Can you work these out from the model? Positions are in its coordinate system, mm. A direction names the side the tool comes from. Give positions to 0.01 mm unless a question says otherwise; leave off trailing zeros. Loops run counter-clockwise (first coordinate to the right, second up) from the corner with the lowest first, then second, coordinate; pieces in that order, holes last. Notation, with made-up numbers: M 21,8.25 L 69,8.25 A26 cw 69,26.25 Z; hole C 48.25,-7.75 d7. An arc over 180 degrees is marked long. Answer as a JSON object with one key per item and string values.
Autodesk Fusion 360 part; units mm, degrees
sketch "Colour Sensor Servo Seat Outline" plane through (0, 0, 0) normal (0, 0, 1) x (1, 0, 0)
  line L0 (0, 0) -> (54.5, 0)
  line L1 (54.5, 0) -> (54.5, 39)
  line L2 (54.5, 39) -> (0, 39)
  line L3 (0, 39) -> (0, 0)
  dimension "d1" = 39
  dimension "d2" = 54.5
extrude "Extrude1" add sketch "Colour Sensor Servo Seat Outline" along normal blind 30
sketch "Colour Sensor Servo Hole" plane through (0, 0, 30) normal (0, 0, 1) x (-1, 0, 0)
  line L0 (0, -39) -> (0, 0)
  line L1 (0, 0) -> (-54.5, 0)
  line L2 (-54.5, 0) -> (-54.5, -39)
  line L3 (-54.5, -39) -> (0, -39)
  line L4 (-54.5, -8.5) -> (-18, -8.5)
  line L5 (-18, -8.5) -> (-18, -21.5)
  line L6 (-18, -21.5) -> (-54.5, -21.5)
  line L7 (-54.5, -21.5) -> (-54.5, -8.5)
  line L8 (-54.5, 0) -> (-18, 0)
  line L9 (-18, 0) -> (-18, -30)
  line L10 (-18, -30) -> (-54.5, -30)
  line L11 (-54.5, -30) -> (-54.5, 0)
  line L12 (-54.5, -21.5) -> (-49.8, -21.5)
  line L13 (-49.8, -21.5) -> (-49.8, -8.5)
  line L14 (-49.8, -8.5) -> (-54.5, -8.5)
  line L15 (-54.5, -8.5) -> (-54.5, -21.5)
  point P0 (-54.5, -21.5)
  point P1 (-54.5, -30)
  dimension "d6" = 13
  dimension "d8" = 36.5
  dimension "d9" = 30
  dimension "d10" = 8.5
  dimension "d11" = 8.5
  dimension "d12" = 4.7
extrude "Extrude2" cut sketch "Colour Sensor Servo Hole" against normal blind 5 contours L2 L4 L6 L7 L11 L12 L13 L14 L15
extrude "Extrude3" cut sketch "Colour Sensor Servo Hole" against normal blind 25.82 contours L4 L5 L6 L9 L13
chamfer "Chamfer1" distance 24 distance2 9 1 edges at (27.25, 39, 0) measured on face at (36.3333, 39, 20)
sketch "Front Ribs" plane through (0, 39, 0) normal (0, 1, 0) x (-1, 0, 0)
  line L0 (-54.5, 24) -> (0, 24)
  line L1 (0, 24) -> (0, 30)
  line L2 (0, 30) -> (-54.5, 30)
  line L3 (-54.5, 30) -> (-54.5, 24)
  line L4 (0, 0) -> (0, 24)
  line L5 (0, 24) -> (-54.5, 24)
  line L6 (-54.5, 24) -> (-54.5, 0)
  line L7 (-54.5, 0) -> (0, 0)
  line L8 (-46, 24) -> (-18, 24)
  line L9 (-18, 24) -> (-18, 0)
  line L10 (-18, 0) -> (-46, 0)
  line L11 (-46, 0) -> (-46, 24)
  line L12 (-18, 24) -> (-9.5, 24)
  line L13 (-9.5, 24) -> (-9.5, 0)
  line L14 (-9.5, 0) -> (-18, 0)
  line L15 (-18, 0) -> (-18, 24)
  dimension "d26" = 8.5
  dimension "d31" = 8.5
  dimension "d39" = 9.5
extrude "Extrude4" cut sketch "Front Ribs" against normal blind 9 contours L0 L5 L7 L8 L9 L10 L11 L15 | L0 L4 L5 L7 L13
chamfer "Chamfer2" distance 24 distance2 9.5 1 edges at (0, 15, 0) measured on face at (0, 10, 18)
sketch "Side Ribs" plane through (0, 0, 0) normal (-1, 0, 0) x (0, -1, 0)
  line L0 (-30, 24) -> (0, 24)
  line L1 (0, 24) -> (0, 30)
  line L2 (0, 30) -> (-39, 30)
  line L3 (-39, 30) -> (-39, 24)
  line L4 (-39, 24) -> (-30, 24)
  line L5 (0, 0) -> (0, 24)
  line L6 (0, 24) -> (-30, 24)
  line L7 (-30, 24) -> (-30, 0)
  line L8 (-30, 0) -> (0, 0)
  line L9 (-21.5, 24) -> (-8.5, 24)
  line L10 (-8.5, 24) -> (-8.5, 0)
  line L11 (-8.5, 0) -> (-21.5, 0)
  line L12 (-21.5, 0) -> (-21.5, 24)
  dimension "d33" = 8.5
  dimension "d34" = 8.5
extrude "Extrude6" cut sketch "Side Ribs" against normal blind 9.5 contours L0 L6 L8 L9 L10 L11 L12
chamfer "Chamfer3" distance 9.5 distance2 9 1 edges at (0, 39, 27) measured on face at (24.1667, 39, 28)
sketch "Servo Cable Hole" plane through (9.5, 0, 0) normal (-1, 0, 0) x (0, -1, 0)
  line L0 (-21.5, 0) -> (-8.5, 0)
  line L1 (-8.5, 0) -> (-8.5, 24)
  line L2 (-8.5, 24) -> (-21.5, 24)
  line L3 (-21.5, 24) -> (-21.5, 0)
  line L4 (-21.5, 0) -> (-21.5, 24)
  line L5 (-21.5, 24) -> (-30, 24)
  line L6 (-30, 24) -> (-30, 0)
  line L7 (-30, 0) -> (-21.5, 0)
  line L8 (-8.5, 24) -> (-8.5, 0)
  line L9 (-8.5, 0) -> (0, 0)
  line L10 (0, 0) -> (0, 24)
  line L11 (0, 24) -> (-8.5, 24)
  line L12 (-21.5, 14.18) -> (-8.5, 14.18)
  line L13 (-8.5, 14.18) -> (-8.5, 4.18)
  line L14 (-8.5, 4.18) -> (-21.5, 4.18)
  line L15 (-21.5, 4.18) -> (-21.5, 14.18)
  dimension "d40" = 10
  dimension "d41" = 4.18
extrude "Extrude7" cut sketch "Servo Cable Hole" against normal blind 8.5 contours L1 L3 L4 L8 L12 L13 L14 L15
equation "d2 = servo_seat_width"
equation "d3 = servo_seat_height"
equation "servo_seat_height = 30 mm"
equation "d6 = servo_hole_width"
equation "servo_hole_width = 13 mm"
equation "d10 = ( 30 mm - servo_hole_width ) / 2"
equation "servo_arm_support_depth = 5 mm"
equation "servo_hole_depth = 25.82 mm"
equation "d19 = servo_seat_height - top_support_thickness"
equation "d20 = 17.50 mm - 8.50 mm"
equation "top_support_thickness = 6 mm"
equation "d22 = -( 17.50 mm - 8.50 mm )"
equation "rib_thickness = 8.5 mm"
equation "d26 = rib_thickness"
equation "d27 = servo_seat_height - top_support_thickness"
equation "d28 = servo_seat_width - 36.50 mm - 8.5 mm"
equation "d31 = rib_thickness"
equation "servo_seat_width = 36.50 mm + 18 mm"
equation "d33 = rib_thickness"
equation "d34 = rib_thickness"
equation "d35 = -( servo_seat_width - 36.50 mm - 8.5 mm )"
equation "d37 = ( servo_seat_width - 36.50 mm - 8.5 mm )"
equation "d39 = ( servo_seat_width - 36.50 mm - 8.5 mm )"
equation "d41 = servo_seat_height - servo_hole_depth"
1) Suppose I cut it at A-A, the plane z = 27.5. Write out the boundary of the cut face in (x, y).
Answer list:
{"outline": "M 0,0 L 54.5,0 L 54.5,8.5 L 18,8.5 L 18,21.5 L 54.5,21.5 L 54.5,39 L 9.5,39 L 0,30 Z"}
2) Suppose I cut it at C-C, the plane x = 24.5. Write out the boundary of the cut face in (y, z), and give its area (3 significant figures).
Answer list:
{"outline": "M 0,0 L 30,0 L 30,24 L 39,24 L 39,30 L 21.5,30 L 21.5,4.18 L 8.5,4.18 L 8.5,30 L 0,30 Z", "area": "618 mm^2"}
3) Please list where these lines run through material, in increasing order: line 1 along Y through (x, z) = (9, 8); line 2 along Y through (x, z) = (35.5, 28.5); line 3 along Z through (x, y) = (17.5, 15.5). Write a range as from..to.
Answer list:
{"line 1": "0..8.5, 21.5..30", "line 2": "0..8.5, 21.5..39", "line 3": "0..4.18, 14.18..30"}
4) Suppose I cut it at B-B, the plane y = 6. Write out the boundary of the cut face in (x, z).
Answer list:
{"outline": "M 0,24 L 9.5,0 L 54.5,0 L 54.5,30 L 0,30 Z"}
5) For faces 1 (the flat face through (5, 15, 24)), 2 (the flat face through (27, 21.5, 15)), 3 (the flat face through (46, 33, 17)), which set-ups out of +Z, -Z, +X, -X, +Y, -Y let a thin tool reach every point of the face, with its end or its side?
Answer list:
{"face 1": "-Z, -X", "face 2": "none", "face 3": "-Z, +Y"}
6) If we mould it in two halves opening along Y, with no side actions, what happens to faces 4 (the flat face through (18, 15, 22)), 5 (the flat face through (27, 0, 15)), 6 (the flat face through (32, 35, 24)), 7 (the flat face through (6, 30, 15))? For each: +Y half, -Y half, draft (parallel to the pull), parting line (faces both ways), or undercut.
Answer list:
{"face 4": "undercut", "face 5": "-Y half", "face 6": "draft", "face 7": "+Y half"}
7) Will these pins go through, and if not, where does the flat tip stop? pin 1 Ø1.3 at (y, z) = (12.5, 2) entering from -X; pin 2 Ø4 at (x, z) = (9, 4.5) entering from +Y; pin 3 Ø9 at (x, z) = (36, 16.5) entering from +Y.
Answer list:
{"pin 1": "x = 9.5", "pin 2": "y = 32.41", "pin 3": "y = 30"}
8) Suppose I cut it at D-D, the plane z = 20.5. Write out the boundary of the cut face in (x, y).
Answer list:
{"outline": "M 1.39,0 L 54.5,0 L 54.5,37.69 L 46,37.69 L 46,30 L 18,30 L 18,37.69 L 9.5,37.69 L 9.5,30 L 1.39,30 L 1.39,21.5 L 9.5,21.5 L 9.5,8.5 L 1.39,8.5 Z; hole M 18,8.5 L 49.8,8.5 L 49.8,21.5 L 18,21.5 Z"}
